from build123d import *

# Parameters (mm, degrees)
SKETCH1_W                                    = 87.86
SKETCH1_H                                    = 44.81
BOSS_EXTRUDE1_DEPTH                          = 2
CSK_FOR_M2_5_COUNTERSUNK_FLAT_HEAD_S_2_COUNT = 2
CSK_FOR_M2_5_COUNTERSUNK_FLAT_HEAD_S_2_PITCH = 31.13
CSK_FOR_M2_5_COUNTERSUNK_FLAT_HEAD_S_3_COUNT = 2
CSK_FOR_M2_5_COUNTERSUNK_FLAT_HEAD_S_3_PITCH = 87.373717444
CSK_FOR_M2_5_COUNTERSUNK_FLAT_HEAD_S_4_COUNT = 2
CSK_FOR_M2_5_COUNTERSUNK_FLAT_HEAD_S_4_PITCH = 81.64
BOSS_EXTRUDE2_DEPTH                          = 15.25
BOSS_EXTRUDE3_DEPTH                          = 15.25
CUT_EXTRUDE1_DEPTH                           = 50
CUT_EXTRUDE1_DEPTH_BACK                      = 15.25
CUT_EXTRUDE4_DEPTH                           = 15.25
SKETCH11_W                                   = 22
SKETCH11_H                                   = 5
CUT_EXTRUDE5_DEPTH                           = 15.25


with BuildPart() as part:
    # Sketch1 → Boss-Extrude1 (new body)
    with BuildSketch(Plane(origin=(0, 0, 0), x_dir=(1, 0, 0), z_dir=(0, 1, 0))):
        Rectangle(SKETCH1_W, SKETCH1_H)
    extrude(amount=BOSS_EXTRUDE1_DEPTH)

    # Sketch3 → CSK for M2.5 Countersunk Flat Head Screw1 (revolve, cut)
    with BuildSketch(Plane(origin=(-40.82, 2, -15.565), x_dir=(0, 0, 1), z_dir=(1, 0, 0))):
        Polygon((0, 0), (0, 2), (1.45, 2), (1.45, 1.3), (2.75, 0), align=None)
    csk_for_m2_5_countersunk_flat_head_screw = revolve(axis=Axis((-40.82, 8.35, -15.565), (0, -1, 0)), mode=Mode.SUBTRACT)

    # CSK for M2.5 Countersunk Flat Head S 2: CSK for M2.5 Countersunk Flat Head Screw1 ×2
    with Locations(*[(0, 0, i * CSK_FOR_M2_5_COUNTERSUNK_FLAT_HEAD_S_2_PITCH) for i in range(1, CSK_FOR_M2_5_COUNTERSUNK_FLAT_HEAD_S_2_COUNT)]):
        add(csk_for_m2_5_countersunk_flat_head_screw, mode=Mode.SUBTRACT)

    # CSK for M2.5 Countersunk Flat Head S 3: CSK for M2.5 Countersunk Flat Head Screw1 ×2
    with Locations(*[Vector(0.9343770917408808, 0, 0.35628563040046085) * (i * CSK_FOR_M2_5_COUNTERSUNK_FLAT_HEAD_S_3_PITCH) for i in range(1, CSK_FOR_M2_5_COUNTERSUNK_FLAT_HEAD_S_3_COUNT)]):
        add(csk_for_m2_5_countersunk_flat_head_screw, mode=Mode.SUBTRACT)

    # CSK for M2.5 Countersunk Flat Head S 4: CSK for M2.5 Countersunk Flat Head Screw1 ×2
    with Locations(*[(i * CSK_FOR_M2_5_COUNTERSUNK_FLAT_HEAD_S_4_PITCH, 0, 0) for i in range(1, CSK_FOR_M2_5_COUNTERSUNK_FLAT_HEAD_S_4_COUNT)]):
        add(csk_for_m2_5_countersunk_flat_head_screw, mode=Mode.SUBTRACT)

    # Sketch5 → Boss-Extrude2 (add)
    with BuildSketch(Plane(origin=(0, 2, 0), x_dir=(1, 0, 0), z_dir=(0, 1, 0))):
        Polygon((-38.07, 15.565), (-38.07, 22.405), (-36.87, 22.405), (-36.87, -22.405), (-38.07, -22.405), align=None)
    extrude(amount=BOSS_EXTRUDE2_DEPTH)

    # Sketch6 → Boss-Extrude3 (add)
    with BuildSketch(Plane(origin=(0, 2, 0), x_dir=(1, 0, 0), z_dir=(0, 1, 0))):
        Polygon((-36.87, 22.405), (38.07, 22.405), (38.07, -22.405), (-36.87, -22.405), (-36.87, -21.205), (36.87, -21.205), (36.87, 21.205), (-36.87, 21.205), align=None)
    extrude(amount=BOSS_EXTRUDE3_DEPTH)

    # Sketch7 → Cut-Extrude1 (cut, two sides: drawn at the far end of the back side and taken through both)
    with BuildSketch(Plane.XY.offset(-21.205).offset(-CUT_EXTRUDE1_DEPTH_BACK)):
        Polygon((0, 2), (-11, 2), (-11, 6), (11, 6), (11, 2), align=None)
    extrude(amount=CUT_EXTRUDE1_DEPTH + CUT_EXTRUDE1_DEPTH_BACK, mode=Mode.SUBTRACT)

    # Sketch10 → Cut-Extrude4 (cut)
    with BuildSketch(Plane(origin=(0, 2, 0), x_dir=(1, 0, 0), z_dir=(0, 1, 0))):
        Polygon((-11, 21.205), (-11, 22.405), (11, 22.405), (11, 17.405), (-11, 17.405), align=None)
    extrude(amount=-CUT_EXTRUDE4_DEPTH, mode=Mode.SUBTRACT)

    # Sketch11 → Cut-Extrude5 (cut)
    with BuildSketch(Plane(origin=(0, 2, 0), x_dir=(1, 0, 0), z_dir=(0, 1, 0))):
        with Locations((0, -19.905)):
            Rectangle(SKETCH11_W, SKETCH11_H)
    extrude(amount=-CUT_EXTRUDE5_DEPTH, mode=Mode.SUBTRACT)


solid = part.part
Can you work these out from the model? Positions are in its coordinate system, mm. A direction names the side the tool comes from. Give positions to 0.01 mm unless a question says otherwise; leave off trailing zeros. Loops run counter-clockwise (first coordinate to the right, second up) from the corner with the lowest first, then second, coordinate; pieces in that order, holes last. Notation, with made-up numbers: M -29,-28 L -1,-28 A20 ccw -1,-24 Z; hole C 70,-29 d9. An arc over 180 degrees is marked long. One line per item, written item: value. Start each with the question number.
1) Thinking about a two-plate mould opening in X: for faces 5 (the face through (-41, 2, 0)), 6 (the face through (11, 1.7, -20.5)), 7 (the face through (43.93, 1, 0)), which applies, +X half, -X half, draft (parallel to the pull), parting line (faces both ways), or undercut?
2) If we section it at A-A, the plane x = -40.82: Write out the boundary of the cut face in (y, z) (3 decimals), and give its area (3 significant figures).
3) If I drill on line 1 (Z direction, x = -40.82, y = 0.3) (3 decimals); line 2 (Z direction, x = -2, y = 6.5) (3 decimals); line 3 (X direction, y = 11.5, z = 13), over which ranges is the centre line in solid material (lowest first)? Write a range as [from, to].
4) If we section it at B-B, the plane y = 3: Write out the boundary of the cut face in (x, z) (3 decimals), and give its area (3 significant figures).
5) If we section it at D-D, the plane x = -32: Write out the boundary of the cut face in (y, z) (3 decimals), and give its area (3 significant figures).
6) On a 3-axis mill with a long thin cutter (end or side, diameter ignored), from which of +Z, -Z, +X, -X, +Y, -Y can I reach the whole of each face in a straight line? I mean faces 1 (the face through (-36.87, 10, 0)), 2 (the face through (-11, 1.7, -20.5)), 3 (the face through (0, 1, 17.405)), 4 (the face through (0, 1, -17.405)). Say none if no direction works.
7) I'm going to push flat-ended pins straight in: pin 1 (10 mm diameter, centred on y = 14, z = 9.5, fed in from +X); pin 2 (1 mm diameter, centred on x = 0.5, z = 22, fed in from -Y); pin 3 (5 mm diameter, centred on y = 7, z = 2, fed in from -X). Where does each tip first touch, or does it pass through?
8) If we section it at C-C, the plane y = 13.75: Write out the boundary of the cut face in (x, z) (3 decimals), and give its area (3 significant figures).
Completed:
1. face 5: draft
1. face 6: undercut
1. face 7: +X half
2. outline: M 0,-22.405 L 2,-22.405 L 2,-18.315 L 0.7,-17.015 L 0,-17.015 Z; M 0,-14.115 L 0.7,-14.115 L 2,-12.815 L 2,12.815 L 0.7,14.115 L 0,14.115 Z; M 0,17.015 L 0.7,17.015 L 2,18.315 L 2,22.405 L 0,22.405 Z
2. area: 74.6 mm^2
3. line 1: z = [-22.405, -17.015], [-14.115, 14.115], [17.015, 22.405]
3. line 2: z = [-22.405, -21.205], [21.205, 22.405]
3. line 3: x = [-38.07, -36.87], [36.87, 38.07]
4. outline: M -38.07,-22.405 L -11,-22.405 L -11,-21.205 L -36.87,-21.205 L -36.87,21.205 L -11,21.205 L -11,22.405 L -38.07,22.405 Z; M 11,-22.405 L 38.07,-22.405 L 38.07,22.405 L 11,22.405 L 11,21.205 L 36.87,21.205 L 36.87,-21.205 L 11,-21.205 Z
4. area: 232 mm^2
5. outline: M 0,-22.405 L 17.25,-22.405 L 17.25,-21.205 L 2,-21.205 L 2,21.205 L 17.25,21.205 L 17.25,22.405 L 0,22.405 Z
5. area: 126 mm^2
6. face 1: +Y
6. face 2: -Z, -Y
6. face 3: +Z, +Y, -Y
6. face 4: -Z, +Y, -Y
7. pin 1: stops at x = 38.07
7. pin 2: stops at y = 6
7. pin 3: stops at x = -38.07
8. outline: M -38.07,-22.405 L 38.07,-22.405 L 38.07,22.405 L -38.07,22.405 Z; hole M -36.87,-21.205 L 36.87,-21.205 L 36.87,21.205 L -36.87,21.205 Z
8. area: 285 mm^2
